from build123d import *

# Parameters (mm, degrees)
SKETCH1_W           = 21.59
SKETCH1_H           = 26.222681286
SKETCH1_R           = 3.175
BOSS_EXTRUDE1_DEPTH = 22.098
BOSS_EXTRUDE2_DEPTH = 5.588


with BuildPart() as part:
    # Sketch1 → Boss-Extrude1 (new body)
    with BuildSketch(Plane.XY):
        with Locations((439.785229177, 122.101713944)):
            Rectangle(SKETCH1_W, SKETCH1_H)
        with Locations(Location((437.331098026, 130.5, 0), (0, 0, 180))):
            Circle(SKETCH1_R, mode=Mode.SUBTRACT)
        with Locations(Location((437.164813366, 120.5, 0), (0, 0, 180))):
            Circle(SKETCH1_R, mode=Mode.SUBTRACT)
    extrude(amount=BOSS_EXTRUDE1_DEPTH)

    # Sketch2 → Boss-Extrude2 (add)
    with BuildSketch(Plane(origin=(0, 108.990373301, 0), x_dir=(1, 0, 0), z_dir=(0, 1, 0))):
        Polygon((428.662736998, -43.850251272), (440.571529023, 23.68786443), (461.83352841, 19.938800274), (449.924736386, -47.599315428), align=None)
    extrude(amount=-BOSS_EXTRUDE2_DEPTH)


solid = part.part
Read the model definition and answer for the solid it produces. Units are mm, in the model's axes. A direction names the side the tool comes from. Round coordinates to 2 decimals unless told otherwise and drop trailing zeros. Loops run counter-clockwise (first coordinate to the right, second up) from the corner with the lowest first, then second, coordinate; pieces in that order, holes last. Notation, with made-up numbers: (-30, 68.25) - (4, 68.25) arc R4 cw to (4, 73.25) - close; hole circle Ø2 at (-21.5, 64). An arc over 180 degrees is marked (long way). One line per question, with ' | ' between items. Start each with the question number.
Q1. Section A-A on y = 130.5 is taken. Give the vertices of the cut face in (x, z), plus the area to 3 significant figures.
Q2. Section C-C on x = 448 is taken. Give the vertices of the cut face in (y, z), plus the area to 3 significant figures.
Q3. Section D-D on y = 106.5 is taken. Give the vertices of the cut face in (x, z).
Q4. Find the intervals of material crossed by L1, parallel to X at y = 120.5, z = 16.25; L2, parallel to X at y = 130.5, z = 16.75; L3, parallel to Y at x = 441.5, z = -16, in increasing order.
Q5. For faces 1 (the flat face through (442, 122, 0)), 2 (the flat face through (442, 122, 22.098)), 3 (the flat face through (432, 108.99, 11)), 4 (the flat face through (450.58, 122, 11)), determine the directions among +Z, -Z, +X, -X, +Y, -Y from which every point of the face is accessible in a straight line to the end or side of a thin tool.
Q6. For a pull along X with two mould halves and no side action, classify faces 5 (the cylindrical face through (435.624, 127.823, 10.894)), 6 (the flat face through (445, 103.402, 11)), 7 (the cylindrical face through (439.5, 118.35, 10.89)), 8 (the flat face through (451.05, 106.24, -21.84)) as +X half, -X half, draft (parallel to the pull), parting line (faces both ways), or undercut.
Q7. Flat-ended cylindrical pins translate along their axes: pin 1 (8 mm diameter, centred on x = 435, y = 115, fed in from -Z); pin 2 (6.5 mm diameter, centred on x = 438.5, y = 116.5, fed in from +Z); pin 3 (5 mm diameter, centred on x = 445, z = 32.5, fed in from +Y). Find the tip coordinate at first contact, or state that the pin passes through.
Q8. Section B-B on z = 20 is taken. Give the vertices of the cut face in (x, y) (3 decimals), plus the area to 3 significant figures.
Established:
1) outline: (428.99, 0) - (434.16, 0) - (434.16, 22.1) - (428.99, 22.1) - close; (440.51, 0) - (450.58, 0) - (450.58, 22.1) - (440.51, 22.1) - close | area: 337 mm²
2) outline: (103.4, -22.38) - (108.99, -22.38) - (108.99, 0) - (135.21, 0) - (135.21, 22.1) - (108.99, 22.1) - (108.99, 47.26) - (103.4, 47.26) - close | area: 969 mm²
3) outline: (428.66, 43.85) - (440.57, -23.69) - (461.83, -19.94) - (449.92, 47.6) - close
4) L1: 428.99 to 433.99, 440.34 to 450.58 | L2: 428.99 to 434.16, 440.51 to 450.58 | L3: 103.4 to 108.99
5) face 1: -Z, +X, -X, +Y | face 2: +Z, +X, -X, +Y | face 3: -Z, -X, -Y | face 4: +Z, -Z, +X, +Y
6) face 5: undercut | face 6: draft | face 7: undercut | face 8: +X half
7) pin 1: z = 0 | pin 2: z = 22.1 | pin 3: y = 108.99
8) outline: (428.99, 108.99) - (432.868, 108.99) - (432.868, 103.402) - (454.791, 103.402) - (454.791, 108.99) - (450.58, 108.99) - (450.58, 135.213) - (428.99, 135.213) - close; hole circle Ø6.35 at (437.165, 120.5); hole circle Ø6.35 at (437.331, 130.5) | area: 625 mm²
